Check sheet for the modelled part. Datum: model origin and axes. Units: mm. A direction names the side the tool comes from. Coordinates: 2 decimals unless noted, no trailing zeros. Loops run counter-clockwise (first coordinate to the right, second up) from the corner with the lowest first, then second, coordinate; pieces in that order, holes last. Notation, with made-up numbers: M 46.5,68 L 70.5,68 A24 cw 70.5,95 Z; hole C 64.5,-14 d10. An arc over 180 degrees is marked long. Answer in a Markdown table with one row per item. Add a question column.
```python
from build123d import *

# Parameters (mm, degrees)
F0_W      = 101.6
F0_H      = 76.2
F1_DEPTH  = 12.7
F2_W      = 50.8
F2_H      = 25.4
F3_DEPTH  = 4.064
F5_DEPTH  = 50.8
F7_DEPTH  = 50.8
F9_DEPTH  = 50.8
F10_W     = 12.7
F10_H     = 101.6
F11_DEPTH = 6.35
F12_W     = 12.7
F12_H     = 101.6
F13_DEPTH = 6.35


with BuildPart() as f1:
    # F0 (on Front) → F1 (new body)
    with BuildSketch(Plane.XZ):
        with Locations((50.8, 38.1)):
            Rectangle(F0_W, F0_H)
    extrude(amount=F1_DEPTH)

    # F2 (on face) → F3 (join)
    with BuildSketch(Plane.XZ.offset(12.7)):
        with Locations((50.8, 12.7)):
            Rectangle(F2_W, F2_H)
    extrude(amount=F3_DEPTH)

    # F4 (on face) → F5 (join)
    with BuildSketch(Plane.YZ.offset(76.2)):
        Polygon((-20.6267049946, -1.2631730384), (-16.764, 0), (-24.6588314903, 24.1419062159), (-28.5215364849, 22.8787331775), align=None)
    extrude(amount=-F5_DEPTH)

    # F6 (on face) → F7 (join)
    with BuildSketch(Plane.YZ.offset(76.2)):
        with BuildLine():
            Line((-16.5507770221, 0), (-16.764, 0))
            ThreePointArc((-16.764, 0), (-17.5513062441, -2.2836680049), (-15.3387688414, -1.31430279))
            ThreePointArc((-15.3387688414, -1.31430279), (-15.6880232962, -0.4203850569), (-16.5507770221, 0))
        make_face()
        with BuildLine():
            ThreePointArc((-16.5507770221, 0), (-16.6573885111, 0.0043168797), (-16.764, 0))
            Line((-16.764, 0), (-16.5507770221, 0))
        make_face()
    extrude(amount=-F7_DEPTH)

    # F8 (on face) → F9 (join)
    with BuildSketch(Plane.YZ.offset(76.2)):
        with BuildLine():
            Line((-20.6267049946, -1.2631730384), (-28.5215364849, 22.8787331775))
            Line((-28.5215364849, 22.8787331775), (-52.1061010659, 49.1076633334))
            ThreePointArc((-52.1061010659, 49.1076633334), (-60.3932888084, 49.3824101727), (-60.6419928372, 41.0943999887))
            Line((-60.6419928372, 41.0943999887), (-20.6267049946, -1.2631730384))
        make_face()
    extrude(amount=-F9_DEPTH)

    # F10 (on face) → F11 (join)
    with BuildSketch(Plane(origin=(0, 0, 0), x_dir=(1, 0, 0), z_dir=(0, 0, -1))):
        with Locations((88.9, 6.0887979344)):
            Rectangle(F10_W, F10_H)
    extrude(amount=F11_DEPTH)

    # F12 (on face) → F13 (join)
    with BuildSketch(Plane(origin=(0, 0, 0), x_dir=(1, 0, 0), z_dir=(0, 0, -1))):
        with Locations((12.7, 6.8910890259)):
            Rectangle(F12_W, F12_H)
    extrude(amount=F13_DEPTH)


solid = f1.part
```
Q1. Cross-section at D-D (y = -9.5). Record the cut outline in (x, z), plus the area to 3 significant figures.
Q2. Thickness scan on L1, parallel to Z at x = 6.5, y = 16; L2, parallel to Y at x = 39.5, z = 13; L3, parallel to Y at x = 70.5, z = 19.5. Record the ranges inside material, lowest first.
Q3. Cross-section at B-B (z = 14.5). Record the cut outline in (x, y).
Q4. Access from +Z, -Z, +X, -X, +Y, -Y to the whole of each face (thin tool, end or side, straight path). Record for faces 5 (the face through (50, 0, 39)), 6 (the face through (13, -36, 0)), 7 (the face through (3, -6, 0)).
Q5. Cross-section at C-C (x = 15.5). Record the cut outline in (y, z).
Q6. Cross-section at A-A (y = 31.5). Record the cut outline in (x, z).
Q7. Go/stop test with flat-tipped pins: pin 1 (1.9 mm diameter, centred on x = 90.5, z = -2, fed in from -Y); pin 2 (3 mm diameter, centred on y = -21.5, z = -2.5, fed in from -X); pin 3 (1.9 mm diameter, centred on y = -7, z = -2, fed in from +X). Record where each tip stops, or that it passes through.
Q8. Mould release check, pull along Y, two halves, no side actions. Record for faces 1 (the face through (50, -12.7, 47)), 2 (the face through (0, -6, 38)), 3 (the face through (89, -56.889, -3)), 4 (the face through (51.16, -40.15, 35.81)): released by +Y, released by -Y, zero draft, split by the parting line, or undercut.
Answer key:
| question | item | result |
|---|---|---|
| 1 | outline | M 0,0 L 6.35,0 L 6.35,-6.35 L 19.05,-6.35 L 19.05,0 L 82.55,0 L 82.55,-6.35 L 95.25,-6.35 L 95.25,0 L 101.6,0 L 101.6,76.2 L 0,76.2 Z |
| 1 | area | 7,900 mm^2 |
| 2 | L1 | -6.35 to 0 |
| 2 | L2 | -34.1 to -21.02, -16.76 to 0 |
| 2 | L3 | -40.24 to -23.14, -16.76 to 0 |
| 3 | outline | M 0,-12.7 L 25.4,-12.7 L 25.4,-16.76 L 76.2,-16.76 L 76.2,-12.7 L 101.6,-12.7 L 101.6,0 L 0,0 Z; M 25.4,-35.52 L 76.2,-35.52 L 76.2,-21.51 L 25.4,-21.51 Z |
| 4 | face 5 | +Z, +X, -X, +Y |
| 4 | face 6 | +Z, -X, -Y |
| 4 | face 7 | -Z, -X, +Y, -Y |
| 5 | outline | M -57.69,-6.35 L 43.91,-6.35 L 43.91,0 L 0,0 L 0,76.2 L -12.7,76.2 L -12.7,0 L -57.69,0 Z |
| 6 | outline | M 6.35,-6.35 L 19.05,-6.35 L 19.05,0 L 6.35,0 Z; M 82.55,-6.35 L 95.25,-6.35 L 95.25,0 L 82.55,0 Z |
| 7 | pin 1 | y = -56.89 |
| 7 | pin 2 | x = 6.35 |
| 7 | pin 3 | x = 95.25 |
| 8 | face 1 | undercut |
| 8 | face 2 | zero draft |
| 8 | face 3 | released by -Y |
| 8 | face 4 | undercut |
